CAD build for the part. Positions are in the model's coordinates, mm. A direction names the side the tool comes from. Give positions to 0.01 mm unless a question says otherwise; leave off trailing zeros. Order: outer loops, then holes, each group sorted by start corner. A loop starts at its lowest first (then second) coordinate and runs counter-clockwise, first axis right, second up.
Item 1: Which spindle directions (+Z, -Z, +X, -X, +Y, -Y) get a long thin tool onto all of the face, cutting with end or side? Do faces 1 (the flat face through (-2, 16, 2)), 2 (the cylindrical face through (5.879, 44.116, 1.622)), 3 (the flat face through (8, 24, 4.5)). Say none if no direction does.
Item 2: Flat gauge pins, fed straight in: P1, Ø1.5, axis at y = 1.5, z = 1, coming from the -X side; P2, Ø2.5, axis at y = 56, z = 1, coming from the +X side; P3, Ø1.2, axis at y = 19, z = 2.5, coming from the +X side; P4, Ø9.5, axis at x = 37.75, y = 41.35, coming from the -Z side. Where does each tip first touch, or does it go through?
Item 3: Two-plate mould, pull along X, no slides. Class faces 4 (the flat face through (6, 29.05, 6)), 5 (the flat face through (25, 57.75, 7)), 6 (the cylindrical face through (-9.13, 34.78, 3.94)): released by +X, released by -X, zero draft, split by the parting line, or undercut.
Item 4: Band-saw the part on C-C on y = 2. Give the cut face in (x, z).
Item 5: Wall check: L1, parallel to X at y = 10.35, z = 0.7; L2, parallel to Y at x = 6.75, z = 6.3; L3, parallel to Y at x = 6.75, z = 2.3. Give the ranges that are in metal, low to high.
Item 6: Band-saw the part on D-D on y = 24. Give the cut face in (x, z), plus the area to 3 significant figures.
Item 7: Band-saw the part on A-A on z = 1.75. Count the separate pieces of the cut face and the enclosed holes in it, plus the area to 3 significant figures.
Autodesk Inventor part; units mm, degrees
ref_plane "YZ Plane" through (0, 0, 0) normal (1, 0, 0) x (0, 1, 0)
ref_plane "XZ Plane" through (0, 0, 0) normal (0, 1, 0) x (-1, 0, 0)
ref_plane "XY Plane" through (0, 0, 0) normal (0, 0, 1) x (1, 0, 0)
sketch "Sketch1" plane through (0, 0, 0) normal (0, 0, 1) x (1, 0, 0)
  line L0 (0, 0) -> (45.5, 0)
  line L1 (45.5, 0) -> (45.5, 54.5)
  line L2 (0, 30.5) -> (-0.25, 30.5)
  line L3 (45.5, 54.5) -> (0, 54.5)
  line L4 (-5.4281, 33.75) -> (-8.7859, 33.3971)
  arc A0 (-9.25, 36.25) -> (-8.7859, 33.3971) centre (-0.25, 36.25) ccw
  arc A1 (-0.25, 57.75) -> (-9.25, 48.75) centre (-0.25, 48.75) ccw
  line L5 (-9.25, 48.75) -> (-9.25, 36.25)
  line L6 (0, 0) -> (0, 3)
  line L7 (0, 3) -> (-3.25, 3)
  line L8 (-3.25, 3) -> (-3.25, 16)
  line L9 (-3.25, 16) -> (0, 16)
  line L10 (0, 16) -> (0, 30.5)
  arc A2 (-5.4281, 33.75) -> (-0.25, 30.5) centre (-0.25, 36.25) ccw
  line L11 (0, 54.5) -> (0, 57.75)
  line L12 (0, 57.75) -> (-0.25, 57.75)
  dimension "d0" = 45.5
  dimension "d1" = 54.5
  dimension "d9" = 84
  dimension "d10" = 13
  dimension "d11" = 3
  dimension "d12" = 3.25
  dimension "d13" = 14.5
  dimension "d18" = 9
  dimension "d19" = 54.75
  dimension "d24" = 12.5
  dimension "d27" = 5.75
  dimension "d30" = 3.25
  dimension "d31" = 45.5
  dimension "d68" = 0.25
  dimension "d69" = 3.25
extrude "Extrusion1" add sketch "Sketch1" along normal blind 4
sketch "Sketch2" plane through (0, 0, 4) normal (0, 0, 1) x (1, 0, 0)
  line L0 (0, 0) -> (45.5, 0)
  line L1 (0, 57.75) -> (-0.25, 57.75)
  arc A0 (-0.25, 57.75) -> (-9.25, 48.75) centre (-0.25, 48.75) ccw
  line L2 (-9.25, 48.75) -> (-9.25, 36.25)
  arc A1 (-9.25, 36.25) -> (-8.7859, 33.3971) centre (-0.25, 36.25) ccw
  arc A2 (-5.4281, 33.75) -> (-0.25, 30.5) centre (-0.25, 36.25) ccw
  line L3 (-3.25, 16) -> (-3.25, 3)
  arc A3 (-9.25, 36.25) -> (-3.25, 27.7647) centre (-0.25, 36.25) ccw
  line L4 (0, 57.75) -> (48.75, 57.75)
  line L5 (48.75, 57.75) -> (48.75, -3.25)
  line L6 (48.75, -3.25) -> (-3.25, -3.25)
  line L7 (-3.25, 27.7647) -> (-3.25, -3.25)
  dimension "d32" = 48.75
  dimension "d33" = 61
extrude "Extrusion2" add sketch "Sketch2" along normal blind 4
sketch "Sketch4" plane through (0, 0, 0) normal (0, 0, -1) x (-1, 0, 0)
  line L0 (-48.75, 57.75) -> (0, 57.75)
  line L1 (-48.75, -3.25) -> (-48.75, 57.75)
  point P0 (-37.75, 41.35)
  point P1 (-6.75, 41.35)
  point P2 (-37.75, 10.35)
  point P3 (-6.75, 10.35)
  dimension "d39" = 31
  dimension "d40" = 31
  dimension "d41" = 16.4
  dimension "d42" = 11
hole "Hole1" at (37.75, 41.35, 0) at (6.75, 41.35, 0) at (37.75, 10.35, 0) at (6.75, 10.35, 0) direction (0, 0, 1) diameter 3 end through all counterbore diameter 5.8 counterbore depth 3.2
sketch "Sketch5" plane through (0, 0, 8) normal (0, 0, 1) x (1, 0, 0)
  circle A0 centre (37.75, 10.35) radius 1.5
  circle A1 centre (37.75, 41.35) radius 1.5
  circle A2 centre (6.75, 41.35) radius 1.5
  circle A3 centre (6.75, 10.35) radius 1.5
  line L0 (6.75, 41.35) -> (37.75, 10.35) construction
  line L1 (37.75, 41.35) -> (6.75, 10.35) construction
  point P0 (0, 0)
  point P1 (22.25, 25.85)
hole "Hole2" at (22.25, 25.85, 8) direction (0, 0, -1) diameter 10 end through all counterbore diameter 22 counterbore depth 2.5
sketch "Sketch6" plane through (0, 0, 0) normal (0, 0, -1) x (-1, 0, 0)
  circle A0 centre (-6.75, 41.35) radius 2.9
  circle A1 centre (-6.75, 10.35) radius 2.9
  circle A2 centre (-35.25, 48.25) radius 2.25
  circle A3 centre (0.75, 40.85) radius 2.25
  circle A4 centre (-5.85, 25.35) radius 2.25
hole "Hole3" at (35.25, 48.25, 0) at (-0.75, 40.85, 0) at (5.85, 25.35, 0) direction (0, 0, 1) diameter 4.5 end through all
sketch "Sketch7" plane through (0, 0, 8) normal (0, 0, 1) x (1, 0, 0)
  circle A0 centre (-0.75, 40.85) radius 2.25
  circle A1 centre (35.25, 48.25) radius 2.25
  circle A2 centre (5.85, 25.35) radius 2.25
  line L0 (3.5224, 40.85) -> (1.3862, 37.15)
  line L1 (1.3862, 37.15) -> (-2.8862, 37.15)
  line L2 (-2.8862, 37.15) -> (-5.0224, 40.85)
  line L3 (-5.0224, 40.85) -> (-2.8862, 44.55)
  line L4 (-2.8862, 44.55) -> (1.3862, 44.55)
  line L5 (1.3862, 44.55) -> (3.5224, 40.85)
  line L6 (39.5224, 48.25) -> (37.3862, 44.55)
  line L7 (37.3862, 44.55) -> (33.1138, 44.55)
  line L8 (33.1138, 44.55) -> (30.9776, 48.25)
  line L9 (30.9776, 48.25) -> (33.1138, 51.95)
  line L10 (33.1138, 51.95) -> (37.3862, 51.95)
  line L11 (37.3862, 51.95) -> (39.5224, 48.25)
  line L12 (10.1224, 25.35) -> (7.9862, 21.65)
  line L13 (7.9862, 21.65) -> (3.7138, 21.65)
  line L14 (3.7138, 21.65) -> (1.5776, 25.35)
  line L15 (1.5776, 25.35) -> (3.7138, 29.05)
  line L16 (3.7138, 29.05) -> (7.9862, 29.05)
  line L17 (7.9862, 29.05) -> (10.1224, 25.35)
  point P0 (0, 0)
  dimension "d64" = 7.4
extrude "Extrusion3" cut sketch "Sketch7" against normal blind 3.5
properties part number "ExtruderSatoerMotorMount"
The answers:
1. face 1: -Z, -X
1. face 2: -Z
1. face 3: +Z
2. P1: stops at x = 0
2. P2: stops at x = 0
2. P3: stops at x = 45.5
2. P4: stops at z = 0
3. face 4: undercut
3. face 5: zero draft
3. face 6: released by -X
4. outline: (-3.25, 4) - (0, 4) - (0, 0) - (45.5, 0) - (45.5, 4) - (48.75, 4) - (48.75, 8) - (-3.25, 8) - close
5. L1: x = -3.25 to 3.85, 9.65 to 34.85, 40.65 to 45.5
5. L2: y = -3.25 to 8.85, 11.85 to 21.65, 29.05 to 39.85, 42.85 to 57.75
5. L3: y = 0 to 7.45, 13.25 to 23.29, 27.41 to 38.45, 44.25 to 54.5
6. outline: (-3.25, 4) - (0, 4) - (0, 0) - (4.05, 0) - (4.05, 4.5) - (2.36, 4.5) - (2.36, 8) - (-3.25, 8) - close; (7.65, 0) - (17.6, 0) - (17.6, 5.5) - (11.41, 5.5) - (11.41, 8) - (9.34, 8) - (9.34, 4.5) - (7.65, 4.5) - close; (26.9, 0) - (45.5, 0) - (45.5, 4) - (48.75, 4) - (48.75, 8) - (33.09, 8) - (33.09, 5.5) - (26.9, 5.5) - close
6. area: 244 mm2
7. separate pieces: 1
7. enclosed holes: 8
7. area: 2,510 mm2
